Design review of the part built by this model. Coordinates are the model's own, in mm. Face numbers are marked on the shaded views. A direction names the side the tool comes from. Round coordinates to 2 decimals unless told otherwise and drop trailing zeros. Write each loop counter-clockwise with the first axis right and the second up, starting at its lowest first coordinate (ties: lowest second). Pieces come first, ordered by that corner, then holes. Notation, with made-up numbers: (49, 72.25) -> (104, 72.25) arc R17 cw to (104, 81.25) -> close; hole circle Ø5 at (57.25, -35.75). An arc over 180 degrees is marked (long way). One line per question, with ' | ' between items. Start each with the question number.
1) Insertion check: pin 1 Ø1.2 at (y, z) = (2, 2) entering from -X; pin 2 Ø1.2 at (y, z) = (5.5, -2) entering from +X; pin 3 Ø0.5 at (x, y) = (1.5, 5.5) entering from +Z. Each pin has a flat end and moves straight along its axis. Give the tip position at first contact, or say it passes through.
2) For the marked faces 1, 2 and 3, list the 3-axis set-ups (+Z, -Z, +X, -X, +Y, -Y) from which the entire face can be reached by the end or side of a thin tool; tool diameter is ignored.
3) Consider section C-C (x = 0). Give the boundary of the cut face in (y, z), then the cut area to 3 significant figures.
4) Consider section A-A (y = 6.75). Give the boundary of the cut face in (x, z).
5) Consider section D-D (z = 1.05). Give the boundary of the cut face in (x, y).
6) Consider section B-B (z = 0). Give the boundary of the cut face in (x, y), then the cut area to 3 significant figures.
7) For probe 1 along X at (y, z) = (4.25, -2.05); probe 2 along Y at (x, z) = (-0.25, 1.6), list the stretches that pass through material, from the lowest coordinate up.
```python
from build123d import *

# Parameters (mm, degrees)
BOSS_EXTRUDE1_DEPTH = 7.62
SKETCH2_R           = 0.82804
BOSS_EXTRUDE2_DEPTH = 7.62


with BuildPart() as part:
    # Sketch1 → Boss-Extrude1 (new body)
    with BuildSketch(Plane(origin=(0, 0, 0), x_dir=(1, 0, 0), z_dir=(0, 1, 0))):
        Polygon((0.8636, 0.8636), (2.413, 0.8636), (2.413, -0.8636), (0.8636, -0.8636), (0.8636, -2.413), (-0.8636, -2.413), (-0.8636, -0.8636), (-2.413, -0.8636), (-2.413, 0.8636), (-0.8636, 0.8636), (-0.8636, 2.413), (0.8636, 2.413), align=None)
    extrude(amount=BOSS_EXTRUDE1_DEPTH)

    # Sketch2 → Boss-Extrude2 (add)
    with BuildSketch(Plane(origin=(0, 7.62, 0), x_dir=(1, 0, 0), z_dir=(0, 1, 0))):
        with Locations(Location((0, 0, 0), (0, 0, 270))):
            Circle(SKETCH2_R)
    extrude(amount=BOSS_EXTRUDE2_DEPTH)


solid = part.part
```
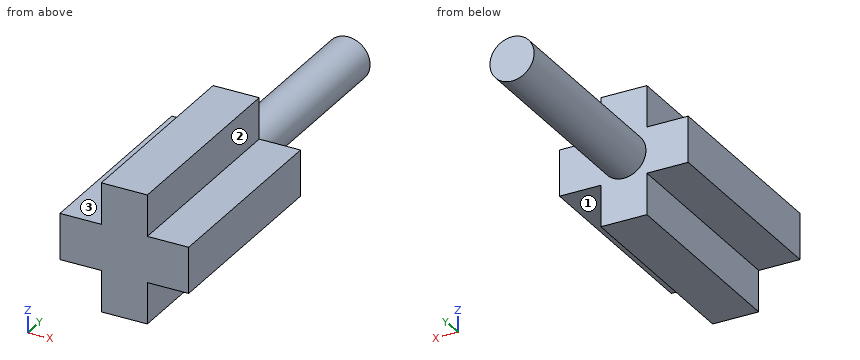
From the geometry:
1) pin 1: stops at x = -0.86 | pin 2: stops at x = 0.86 | pin 3: stops at z = 0.86
2) face 1: -Z, +X, +Y, -Y | face 2: +Z, +X, +Y, -Y | face 3: +Z, -X, +Y, -Y
3) outline: (0, -2.41) -> (7.62, -2.41) -> (7.62, -0.83) -> (15.24, -0.83) -> (15.24, 0.83) -> (7.62, 0.83) -> (7.62, 2.41) -> (0, 2.41) -> close | area: 49.4 mm2
4) outline: (-2.41, -0.86) -> (-0.86, -0.86) -> (-0.86, -2.41) -> (0.86, -2.41) -> (0.86, -0.86) -> (2.41, -0.86) -> (2.41, 0.86) -> (0.86, 0.86) -> (0.86, 2.41) -> (-0.86, 2.41) -> (-0.86, 0.86) -> (-2.41, 0.86) -> close
5) outline: (-0.86, 0) -> (0.86, 0) -> (0.86, 7.62) -> (-0.86, 7.62) -> close
6) outline: (-2.41, 0) -> (2.41, 0) -> (2.41, 7.62) -> (0.83, 7.62) -> (0.83, 15.24) -> (-0.83, 15.24) -> (-0.83, 7.62) -> (-2.41, 7.62) -> close | area: 49.4 mm2
7) probe 1: x = -0.86 to 0.86 | probe 2: y = 0 to 7.62
